Input: part model. Units: mm. Frame: model coordinates. A direction names the side the tool comes from. Round coordinates to 2 decimals unless told otherwise and drop trailing zeros. Order: outer loops, then holes, each group sorted by start corner. A loop starts at its lowest first (then second) coordinate and runs counter-clockwise, first axis right, second up.
Item 1: Mould query, pull axis X, two halves, no side actions, for faces 3 (the flat face through (14, -5, 0)), 4 (the flat face through (16.009, -3.836, 7.549)), 5 (the flat face through (12.88, -0.24, 7.4)). Classes: released by +X, released by -X, zero draft, split by the parting line, or undercut.
Item 2: First-contact query: pin 1 (6 mm diameter, centred on x = -0.5, z = 7.5, fed in from -Y); pin 2 (6 mm diameter, centred on y = -9, z = 2, fed in from -X); pin 3 (1.5 mm diameter, centred on y = -3.5, z = 6.5, fed in from -X); pin 4 (1.5 mm diameter, centred on x = 20, y = -8, fed in from -Z). Flat tips, straight axial feed; report the tip coordinate or a pass-through.
Item 3: Line query: L1, parallel to X at y = -8, z = 3.25; L2, parallel to X at y = -10, z = 10; L3, parallel to Y at x = -1.5, z = 5.5. Output: solid intervals per line, ascending.
Item 4: Cut plane A-A on z = 12. Output: boundary loops of the cut face in (x, y).
Item 5: Reachability of faces 1 (the flat face through (15.1, -6.1, 7.4)), 2 (the cylindrical face through (19.27, -2.867, 4.083)) from +Z, -Z, +X, -X, +Y, -Y: full face, straight path, thin tool, end or side. Return the list, or none.
Item 6: Cut plane C-C on y = -10. Output: boundary loops of the cut face in (x, z).
Item 7: Cut plane D-D on x = 2. Output: boundary loops of the cut face in (y, z).
Item 8: Cut plane B-B on z = 8.25. Output: boundary loops of the cut face in (x, y).
```python
from build123d import *

# Parameters (mm, degrees)
F1_DEPTH    = 15
F2_T1_DEPTH = 86.0591430992
F3_R        = 2
F4_DEPTH    = 16.3887129303
F5_R        = 3.5
F5_R_2      = 2
F6_DEPTH    = 3


# Not quite as in the source:
# - a fillet or chamfer that OpenCascade refuses, or shapes differently, is made with other operations: its cross-section is extruded or revolved along the edge and cut away or added


with BuildPart() as f1:
    # F0 (on Top) → F1 (new body)
    with BuildSketch(Plane.XY):
        Polygon((-12.7344739318, -5.4054634817), (0, 0), (30.5970672007, -12.3620175827), (30.5970672007, -3.3620175827), (-12.7344739318, 4.2785022346), align=None)
    extrude(amount=F1_DEPTH)

    # F2: fillet of radius 13 on 1 edges, made by hand

    # F2_s2 → F2_t1 (cut)
    with BuildSketch(Plane.XY.offset(-35.5295715496)):
        with BuildLine():
            ThreePointArc((-12.7344739318, -5.4054634817), (-6.9533889828, 0.5627654484), (1.2614450775, 1.8106440935))
            Line((1.2614450775, 1.8106440935), (-12.7344739318, 4.2785022346))
            Line((-12.7344739318, 4.2785022346), (-12.7344739318, -5.4054634817))
        make_face()
    extrude(amount=F2_T1_DEPTH, mode=Mode.SUBTRACT)

    # F3 (on face) → F4 (cut, through all)
    with BuildSketch(Plane(origin=(0.3476755995, 1.9717663066, 0), x_dir=(-0.984807753, 0.1736481777, 0), z_dir=(0.1736481777, 0.984807753, 0))):
        with Locations((-18.7160372252, 7.5)):
            Circle(F3_R)
    extrude(amount=-F4_DEPTH, mode=Mode.SUBTRACT)

    # F5 (on face) → F6 (cut)
    with BuildSketch(Plane(origin=(0.3476755995, 1.9717663066, 0), x_dir=(-0.984807753, 0.1736481777, 0), z_dir=(0.1736481777, 0.984807753, 0))):
        with Locations((-18.7160372252, 7.5)):
            Circle(F5_R)
        with Locations((-18.7160372252, 7.5)):
            Circle(F5_R_2, mode=Mode.SUBTRACT)
    extrude(amount=-F6_DEPTH, mode=Mode.SUBTRACT)


solid = f1.part
```
From the geometry:
1. face 3: zero draft
1. face 4: undercut
1. face 5: released by +X
2. pin 1: stops at y = -1.49
2. pin 2: stops at x = 14.85
2. pin 3: stops at x = -12.11
2. pin 4: stops at z = 0
3. L1: x = 19.8 to 30.6
3. L2: x = 24.75 to 30.6
3. L3: y = -0.64 to 2
4. outline: (-12.73, -5.41) - (0, 0) - (30.6, -12.36) - (30.6, -3.36) - (1.26, 1.81) arc R13 ccw to start
5. face 1: +Z, -Z, -Y
5. face 2: none
6. outline: (24.75, 0) - (30.6, 0) - (30.6, 15) - (24.75, 15) - close
7. outline: (-0.81, 0) - (1.68, 0) - (1.68, 15) - (-0.81, 15) - close
8. outline: (-12.73, -5.41) - (0, 0) - (15.98, -6.46) - (16.43, -3.91) - (14.89, -3.64) - (15.41, -0.68) - (1.26, 1.81) arc R13 ccw to start; (19.5, -7.88) - (30.6, -12.36) - (30.6, -3.36) - (22.15, -1.87) - (21.63, -4.83) - (20.08, -4.55) - close
